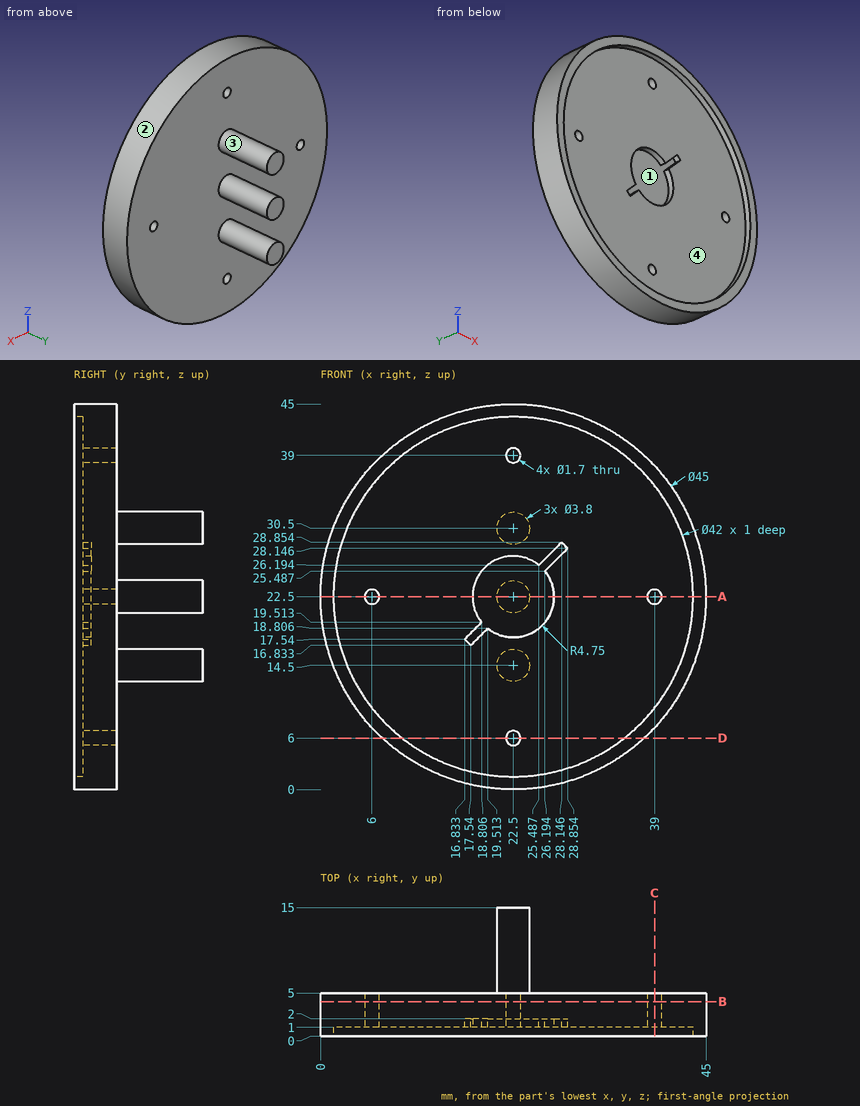
Design review of the part shown in the three views and the two pictorial views. Dimensions are in mm from the part's minimum x, y and z. A direction names the side the tool comes from. Coordinates: 2 decimals unless noted, no trailing zeros. Loops run counter-clockwise (first coordinate to the right, second up) from the corner with the lowest first, then second, coordinate; pieces in that order, holes last. Notation, with made-up numbers: (43.25, 21.25) - (99.25, 21.25) arc R25 ccw to (99.25, 60.25) - close; hole circle Ø2 at (82, 34.25). An arc over 180 degrees is marked (long way). Use a Markdown table: item, result. Add a question column.
Item 1: Mouldability with a two-part tool opening along Z and no side actions: class the marked faces 1 and 2 as pulls with the +Z half, pulls with the -Z half, needs draft (parallel to the pull), parting line crosses it, or undercut.
Item 2: We need section D-D (z = 6). Give the boundary of the cut face in (x, y).
Item 3: For line 1 (Z direction, x = 22.5, y = 0.75); line 2 (Y direction, x = 18.5, z = 23); line 3 (Y direction, x = 29.5, z = 5), list the stretches that pass through material, from the lowest coordinate up.
Item 4: Tool access review of the marked faces 3 and 4: name each direction out of +Z, -Z, +X, -X, +Y, -Y from which nothing blocks a thin tool from reaching the whole face with its end or side.
Item 5: We need section B-B (y = 4). Give the boundary of the cut face in (x, z), and give its area (3 significant figures).
Item 6: We need section C-C (x = 39). Give the boundary of the cut face in (y, z).
Item 7: Insertion check: pin 1 Ø1.5 at (x, y) = (32.5, 5) entering from -Z; pin 2 Ø1.5 at (x, z) = (13, 27) entering from +Y; pin 3 Ø1.5 at (y, z) = (8, 19) entering from -X; pin 4 Ø1 at (x, z) = (9, 25) entering from -Y. Each pin has a flat end and moves straight along its axis. Give the tip position at first contact, or say it passes through.
Item 8: We need section A-A (z = 22.5). Give the boundary of the cut face in (x, y), and give its area (3 significant figures).
Results list:
| question | item | result |
|---|---|---|
| 1 | face 1 | undercut |
| 1 | face 2 | parting line crosses it |
| 2 | outline | (7.2, 0) - (9.51, 0) - (9.51, 1) - (21.65, 1) - (21.65, 5) - (7.2, 5) - close; (23.35, 1) - (35.49, 1) - (35.49, 0) - (37.8, 0) - (37.8, 5) - (23.35, 5) - close |
| 3 | line 1 | z = 0 to 1.5, 43.5 to 45 |
| 3 | line 2 | y = 2 to 5 |
| 3 | line 3 | y = 1 to 5 |
| 4 | face 3 | +Y |
| 4 | face 4 | -Y |
| 5 | outline | circle Ø45 at (22.5, 22.5); hole circle Ø1.7 at (6, 22.5); hole circle Ø1.7 at (22.5, 6); hole circle Ø1.7 at (22.5, 39); hole circle Ø1.7 at (39, 22.5) |
| 5 | area | 1,580 mm^2 |
| 6 | outline | (0, 7.2) - (5, 7.2) - (5, 21.65) - (1, 21.65) - (1, 9.51) - (0, 9.51) - close; (0, 35.49) - (1, 35.49) - (1, 23.35) - (5, 23.35) - (5, 37.8) - (0, 37.8) - close |
| 7 | pin 1 | stops at z = 1.99 |
| 7 | pin 2 | stops at y = 5 |
| 7 | pin 3 | passes through |
| 7 | pin 4 | stops at y = 1 |
| 8 | outline | (0, 0) - (1.5, 0) - (1.5, 1) - (5.15, 1) - (5.15, 5) - (0, 5) - close; (6.85, 1) - (17.75, 1) - (17.75, 2) - (27.25, 2) - (27.25, 1) - (38.15, 1) - (38.15, 5) - (24.4, 5) - (24.4, 15) - (20.6, 15) - (20.6, 5) - (6.85, 5) - close; (39.85, 1) - (43.5, 1) - (43.5, 0) - (45, 0) - (45, 5) - (39.85, 5) - close |
| 8 | area | 198 mm^2 |
